Here's how the part is built. I have some questions about the finished solid (model axes, mm). Round coordinates to 2 decimals unless told otherwise and drop trailing zeros. Loops run counter-clockwise (first coordinate to the right, second up) from the corner with the lowest first, then second, coordinate; pieces in that order, holes last. Notation, with made-up numbers: M 17,9 L 39,9 A14 ccw 39,20 Z; hole C 51,-29.75 d4. An arc over 180 degrees is marked long. Write item = value, one per line. Start each with the question number.
from build123d import *

# Parameters (mm, degrees)
BOSS_EXTRUDE1_DEPTH = 10
CUT_EXTRUDE34_DEPTH = 10


with BuildPart() as part:
    # Sketch1 → Boss-Extrude1 (new body)
    with BuildSketch(Plane.XY):
        with BuildLine():
            Line((-50, 60), (50, 60))
            ThreePointArc((50, 60), (57.071067812, 57.071067812), (60, 50))
            Line((60, 50), (60, -50))
            ThreePointArc((60, -50), (57.071067812, -57.071067812), (50, -60))
            Line((50, -60), (-50, -60))
            ThreePointArc((-50, -60), (-57.071067812, -57.071067812), (-60, -50))
            Line((-60, -50), (-60, 50))
            ThreePointArc((-60, 50), (-57.071067812, 57.071067812), (-50, 60))
        make_face()
    extrude(amount=BOSS_EXTRUDE1_DEPTH)

    # Sketch2 → Cut-Extrude34 (cut)
    with BuildSketch(Plane.XY.offset(10)):
        with BuildLine():
            Line((-31.75, 50), (-14.25, 50))
            Line((-14.25, 50), (-14.25, -13.4375))
            add(Edge.make_bspline(
                [(-14.25, -13.4375), (-14.249048436, -14.095192485), (-14.247210501, -15.365518725), (-14.155202495, -17.18802097), (-14.071008825, -18.863282124), (-13.919099547, -20.389468135), (-13.694677475, -21.767231851), (-13.477363681, -23.005423537), (-13.183250949, -24.081874769), (-12.741246534, -25.307158094), (-12.060262829, -26.683830835), (-10.947573238, -28.118630748), (-9.663624637, -29.428093921), (-8.124738289, -30.518041453), (-6.395166126, -31.399710765), (-4.484411381, -32.052930153), (-2.395167537, -32.416033402), (-0.950570024, -32.471467764), (-0.20703125, -32.5)],
                knots=[0, 0, 0, 0, 1.155499968, 2.231836252, 3.205919964, 4.102923608, 4.924856345, 5.658536265, 6.31071849, 6.882491295, 7.94666036, 8.992281882, 10.060072772, 11.158554251, 12.289267114, 13.461410017, 14.693379945, 16, 16, 16, 16], degree=3))
            add(Edge.make_bspline(
                [(-0.20703125, -32.5), (0.58288694, -32.476949616), (2.123093674, -32.432005269), (4.338435864, -31.990827854), (6.390962967, -31.288322317), (8.237215984, -30.285667879), (9.875357596, -29.083810814), (11.262010144, -27.713317134), (12.356351241, -26.171453388), (13.069602054, -24.748966669), (13.470057261, -23.439691518), (13.770218387, -22.269903853), (13.990269699, -20.8896702), (14.189907481, -19.320545885), (14.309874409, -17.5462778), (14.439958985, -15.58113484), (14.487636189, -13.411670971), (14.495762421, -11.901032563), (14.5, -11.11328125)],
                knots=[0, 0, 0, 0, 1.261321664, 2.459363699, 3.594844139, 4.716940403, 5.803436589, 6.833651888, 7.818396249, 8.814403945, 9.360733334, 10.004355033, 10.743453831, 11.592799886, 12.532235708, 13.585170094, 14.740740724, 16, 16, 16, 16], degree=3))
            Line((14.5, -11.11328125), (14.5, 50))
            Line((14.5, 50), (32, 50))
            Line((32, 50), (32, -8.1640625))
            add(Edge.make_bspline(
                [(32, -8.1640625), (31.997569807, -9.342463626), (31.992896783, -11.608414067), (31.921133218, -14.86474431), (31.768361569, -17.838879649), (31.640051007, -20.531689117), (31.391726127, -22.939545056), (31.133029856, -25.072729698), (30.803299203, -26.923683518), (30.312679818, -29.030769504), (29.466016005, -31.45700185), (28.101082939, -34.250703218), (26.368388756, -36.985906082), (24.320430824, -39.632521321), (22.008098987, -42.091141586), (19.48266259, -44.249491939), (16.78424454, -46.075223595), (13.884648303, -47.523695215), (10.786341582, -48.653393883), (7.458668947, -49.412494488), (3.903899606, -49.925352385), (1.448553234, -49.974618698), (0.18359375, -50)],
                knots=[0, 0, 0, 0, 1.170808336, 2.251350247, 3.235597562, 4.129743112, 4.929140599, 5.639994148, 6.264258765, 6.79612947, 7.788252245, 8.809469599, 9.879094798, 10.999557536, 12.129761673, 13.226370002, 14.293821979, 15.358369427, 16.438775801, 17.562147481, 18.744053101, 20, 20, 20, 20], degree=3))
            add(Edge.make_bspline(
                [(0.18359375, -50), (-0.656870496, -49.98584349), (-2.315089212, -49.957912986), (-4.753790735, -49.711638896), (-7.111274811, -49.34872349), (-9.383111744, -48.819267286), (-11.577186656, -48.13530876), (-13.692916631, -47.293403446), (-15.722439107, -46.298247386), (-17.65439716, -45.158993863), (-19.486413351, -43.927087294), (-21.160781583, -42.561467005), (-22.735120796, -41.163125773), (-24.163948989, -39.673215464), (-25.457997932, -38.107377594), (-26.614602531, -36.462063463), (-27.632044456, -34.737419211), (-28.535916899, -32.902358231), (-29.309543493, -30.863610995), (-29.961739774, -28.548658425), (-30.531513794, -25.921215951), (-30.954936225, -22.975364085), (-31.338813488, -19.720812027), (-31.581786631, -16.149081171), (-31.708896819, -12.260069041), (-31.735952739, -9.563897555), (-31.75, -8.1640625)],
                knots=[0, 0, 0, 0, 1.001158378, 1.975264943, 2.917723546, 3.841610987, 4.75185031, 5.653588123, 6.552117133, 7.442167995, 8.324307438, 9.179605724, 10.014504199, 10.831958861, 11.636465792, 12.43274043, 13.225645099, 14.020104002, 14.867201867, 15.819789774, 16.883317127, 18.068162734, 19.364263498, 20.787406516, 22.332041935, 24, 24, 24, 24], degree=3))
            Line((-31.75, -8.1640625), (-31.75, 50))
        make_face()
    extrude(amount=-CUT_EXTRUDE34_DEPTH, mode=Mode.SUBTRACT)


solid = part.part
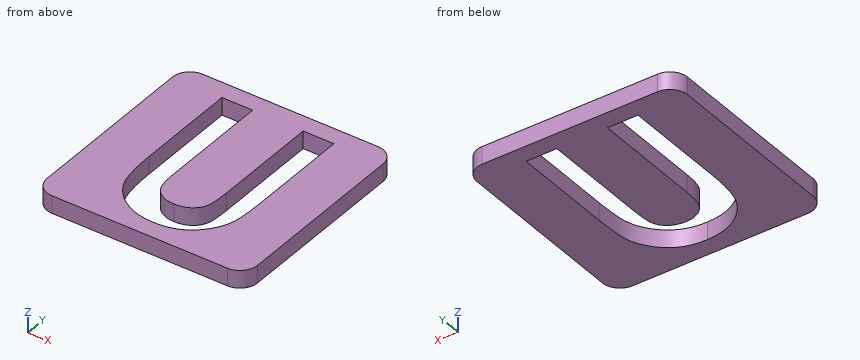
Item 1: I want a section at A-A, the plane y = 41. List the corners of the cut face in (x, z) for me, then the cut area to 3 significant figures.
Item 2: I want a section at B-B, the plane y = -24. State how many separate pieces and enclosed holes the cut face has, then the cut area to 3 significant figures.
Item 3: Please list where these lines run through material, in increasing order: line 1 (X direction, y = 26.5, z = 9.5); line 2 (X direction, y = -45.5, z = 8.5); line 3 (X direction, y = -13, z = 2.5). Write a range as [from, to].
Worked out:
q1.outline = M -60,0 L -31.75,0 L -31.75,10 L -60,10 Z; M -14.25,0 L 14.5,0 L 14.5,10 L -14.25,10 Z; M 32,0 L 60,0 L 60,10 L 32,10 Z
q1.area = 850 mm2
q2.separate_pieces = 3
q2.enclosed_holes = 0
q2.area = 844 mm2
q3.line_1 = [-60, -31.75], [-14.25, 14.5], [32, 60]
q3.line_2 = [-60, -17.06], [17.59, 60]
q3.line_3 = [-60, -31.68], [-14.25, 14.49], [31.96, 60]
